Autodesk Inventor part; units mm, degrees
ref_plane "YZ Plane" through (0, 0, 0) normal (1, 0, 0) x (0, 1, 0)
ref_plane "XZ Plane" through (0, 0, 0) normal (0, 1, 0) x (-1, 0, 0)
ref_plane "XY Plane" through (0, 0, 0) normal (0, 0, 1) x (1, 0, 0)
sketch "Sketch1" plane through (0, 0, 0) normal (0, 1, 0) x (-1, 0, 0)
  line L0 (0, 0) -> (-25.4, 0)
  line L1 (-25.4, 0) -> (-25.4, -25.4)
  line L2 (-25.4, -25.4) -> (0, -25.4)
  line L3 (0, -25.4) -> (0, 0)
  dimension "d0" = 25.4
extrude "Extrusion1" add sketch "Sketch1" along normal blind 6.35
sketch "Sketch2" plane through (0, 6.35, 0) normal (0, 1, 0) x (1, 0, 0)
  circle A0 centre (8.4667, 13.97) radius 0.635
  circle A1 centre (16.9333, 13.97) radius 0.635
  circle A2 centre (16.9333, 11.43) radius 0.635
  circle A3 centre (8.4667, 11.43) radius 0.635
  line L0 (25.4, 0) -> (25.4, 25.4)
  line L1 (0, 0) -> (25.4, 0)
  dimension "d3" = 8.4667
  dimension "d4" = 8.4667
  dimension "d5" = 2.54
  dimension "d6" = 1.27
  dimension "d7" = 11.43
extrude "Extrusion2" cut sketch "Sketch2" against normal blind 6.35
sketch "Sketch4" plane through (0, 0, 0) normal (0, -1, 0) x (1, 0, 0)
  line L0 (25.4, -25.4) -> (0, -25.4)
  arc A0 (9.525, -25.4) -> (15.875, -25.4) centre (12.7, -28.575) ccw
  line L1 (15.875, -25.4) -> (9.525, -25.4)
  point P0 (0, 0)
  dimension "d10" = 90
  dimension "d11" = 6.35
  dimension "d12" = 9.525
extrude "Extrusion3" add sketch "Sketch4" against normal blind 3.175
equation "\"d1\" = 0.25 * d0"
equation "\"d3\" = 0.333333 * d0"
equation "\"d4\" = d3"
equation "\"d8\" = 0.25 * d0"
equation "\"d11\" = 0.25 * d0"
equation "\"d12\" = 0.375 * d0"
equation "\"d13\" = 0.5 * d1"
properties part number "pieceBase"
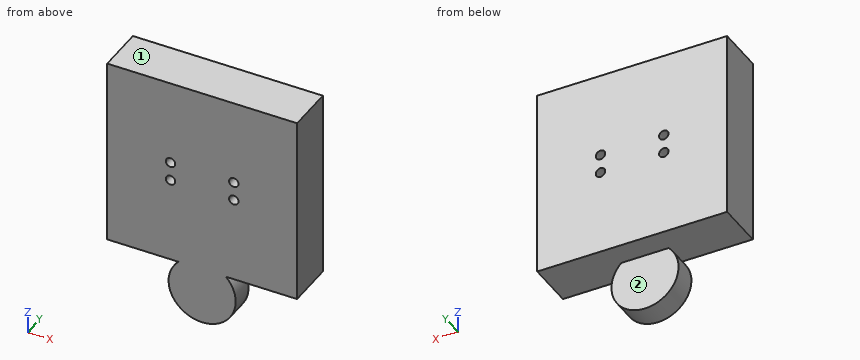
Geometry check sheet. Reference: the model listing, model coordinates, mm. Face numbers are marked on the shaded views. A direction names the side the tool comes from. Round coordinates to 2 decimals unless told otherwise and drop trailing zeros. Order: outer loops, then holes, each group sorted by start corner. A loop starts at its lowest first (then second) coordinate and runs counter-clockwise, first axis right, second up. Notation, with made-up numbers: M -32,42 L 26,42 A12 cw 26,57 Z; hole C 40,88.25 d9. An arc over 180 degrees is marked long. Write each question's results on one line, items separated by ' | '. Start each with the question number.
1. Cross-section at A-A on z = -11.43. Record the boundary of the cut face in (x, y), plus the area to 3 significant figures.
2. Go/stop test with flat-tipped pins: P1, Ø2, axis at x = 13, y = 3, coming from the +Z side; P2, Ø1.1, axis at x = 16.93, z = -11.43, coming from the -Y side; P3, Ø3, axis at x = 11, y = 1, coming from the -Z side. Record where each tip stops, or that it passes through.
3. Material ranges on L1, parallel to X at y = 4, z = -11.43; L2, parallel to Z at x = 9, y = 1.5; L3, parallel to Z at x = 22.25, y = 5.75, recorded low to high. Write a range as from..to.
4. Cross-section at B-B on y = 2.5. Record the boundary of the cut face in (x, z) (3 decimals), plus the area to 3 significant figures.
5. Cross-section at C-C on x = 12.7. Record the boundary of the cut face in (y, z) (3 decimals).
6. Cross-section at D-D on x = 5.25. Record the boundary of the cut face in (y, z).
7. Set-up check for the marked faces 1 and 2: record each of +Z, -Z, +X, -X, +Y, -Y from which the full face is reachable in a straight line by a thin tool's end or side.
Resolved:
1) outline: M 0,0 L 7.83,0 L 7.83,6.35 L 0,6.35 Z; M 9.1,0 L 16.3,0 L 16.3,6.35 L 9.1,6.35 Z; M 17.57,0 L 25.4,0 L 25.4,6.35 L 17.57,6.35 Z | area: 145 mm2
2) P1: z = 0 | P2: through | P3: z = -33.06
3) L1: 0..7.83, 9.1..16.3, 17.57..25.4 | L2: -31.12..-26.03, -25.4..-14.31, -13.63..-11.77, -11.09..0 | L3: -25.4..0
4) outline: M 0,-25.4 L 9.525,-25.4 A4.49 ccw long 15.875,-25.4 L 25.4,-25.4 L 25.4,0 L 0,0 Z; hole C 8.467,-13.97 d1.27; hole C 8.467,-11.43 d1.27; hole C 16.933,-13.97 d1.27; hole C 16.933,-11.43 d1.27 | area: 698 mm2
5) outline: M 0,-33.065 L 3.175,-33.065 L 3.175,-25.4 L 6.35,-25.4 L 6.35,0 L 0,0 Z
6) outline: M 0,-25.4 L 6.35,-25.4 L 6.35,0 L 0,0 Z
7) face 1: +Z, +X, -X, +Y, -Y | face 2: -Z, +X, -X, +Y
